```python
from build123d import *

# Parameters (mm, degrees)
RISER_DEPTH             = 7
SKETCH2_R               = 1.575
MOUNTING_HOLES_DEPTH    = 24.216373532
SKETCH3_W               = 40.15
SKETCH3_H               = 5.15
RECESS_DEPTH            = 3
FLANGE_DEPTH            = 7
SKETCH5_W               = 13.594480272
SKETCH5_H               = 6.925
FLANGE_CUTOUT_DEPTH     = 5
ANGLE_CUTOUT_DEPTH      = 32.901199964
ANGLE_CUTOUT_DEPTH_BACK = 32.901199964
FLANGE_CHAMFER_SIZE     = 1


with BuildPart() as part:
    # Sketch1 → Riser (new body)
    with BuildSketch(Plane(origin=(0, 0, 0), x_dir=(1, 0, 0), z_dir=(0, 1, 0))):
        Polygon((-18.999581839, 7), (18.999581839, 7), (21, 5.75), (21, 0), (-21, 0), (-21, 5.75), align=None)
    extrude(amount=RISER_DEPTH)

    # Sketch2 → Mounting Holes (cut, through all)
    with BuildSketch(Plane.XZ):
        with Locations(Location((16, -3.5, 0), (0, 0, 270))):
            Circle(SKETCH2_R)
        with Locations(Location((-16, -3.5, 0), (0, 0, 90))):
            Circle(SKETCH2_R)
    extrude(amount=-MOUNTING_HOLES_DEPTH, mode=Mode.SUBTRACT)

    # Sketch3 → Recess (cut)
    with BuildSketch(Plane(origin=(0, 7, 0), x_dir=(1, 0, 0), z_dir=(0, 1, 0))):
        with Locations((0, 3.5)):
            Rectangle(SKETCH3_W, SKETCH3_H)
    extrude(amount=-RECESS_DEPTH, mode=Mode.SUBTRACT)

    # Sketch4 → Flange (add)
    with BuildSketch(Plane(origin=(0, 0, 0), x_dir=(1, 0, 0), z_dir=(0, 1, 0))):
        Polygon((-18.999581839, 7), (18.999581839, 7), (7.797240136, 14), (-7.797240136, 14), align=None)
    extrude(amount=FLANGE_DEPTH)

    # Sketch5 → Flange Cutout (cut)
    with BuildSketch(Plane(origin=(0, 7, 0), x_dir=(1, 0, 0), z_dir=(0, 1, 0))):
        with Locations((0, 10.5375)):
            Rectangle(SKETCH5_W, SKETCH5_H)
        Polygon((-18.879556749, 7.075), (-7.797240136, 7.075), (-7.797240136, 14), align=None)
        Polygon((7.797240136, 7.075), (7.797240136, 14), (18.879556749, 7.075), align=None)
    extrude(amount=-FLANGE_CUTOUT_DEPTH, mode=Mode.SUBTRACT)

    # Sketch7 → Angle Cutout (cut, two sides: drawn at the far end of the back side and taken through both)
    with BuildSketch(Plane.ZY.offset(-6.797240136).offset(-ANGLE_CUTOUT_DEPTH_BACK)):
        Polygon((-7.075, 7), (-14, 2), (-14, 7), align=None)
    extrude(amount=ANGLE_CUTOUT_DEPTH + ANGLE_CUTOUT_DEPTH_BACK, mode=Mode.SUBTRACT)

    # Flange Chamfer
    flange_chamfer_edges = [part.edges().sort_by_distance(p)[0] for p in [
        (13.338398442, 2, -7.075),
        (-13.338398442, 2, -7.075),
        (0, 2, -7.075),
    ]]
    chamfer(flange_chamfer_edges, length=FLANGE_CHAMFER_SIZE)


solid = part.part
```
Verification items for the finished model (mm, model axes). A direction names the side the tool comes from. Give positions to 0.01 mm unless a question says otherwise; leave off trailing zeros. Loops run counter-clockwise (first coordinate to the right, second up) from the corner with the lowest first, then second, coordinate; pieces in that order, holes last. Notation, with made-up numbers: M 18.5,63 L 25.5,63 A26 cw 25.5,96 Z; hole C 59,48.25 d1. An arc over 180 degrees is marked long. Return JSON: item names as keys, results as strings.
1) Section check A-A, the plane y = 6. Enter the section's corners in (x, z) (3 decimals), and give its area (3 significant figures).
Findings:
{"outline": "M -21,-5.75 L -18.88,-7.075 L -7.797,-7.075 L -7.797,-8.46 L -6.797,-8.46 L -6.797,-7.075 L 6.797,-7.075 L 6.797,-8.46 L 7.797,-8.46 L 7.797,-7.075 L 18.88,-7.075 L 21,-5.75 L 21,0 L -21,0 Z; hole M -20.075,-6.075 L 20.075,-6.075 L 20.075,-0.925 L -20.075,-0.925 Z", "area": "90.3 mm2"}
2) Gauge pin test, flat ends, axial feed: P1, Ø2.5, axis at y = 3.5, z = -11, coming from the +X side; P2, Ø4, axis at y = 3.5, z = -11, coming from the -X side; P3, Ø4.5, axis at x = 0, z = -11, coming from the +Y side. Record the tip position at first contact, or that the pin passes through.
Findings:
{"P1": "stops at x = 7.8", "P2": "stops at x = -14.72", "P3": "stops at y = 2"}
3) Section check B-B, the plane z = -3.5. Enter the section's corners in (x, y) (3 decimals), and give its area (3 significant figures).
Findings:
{"outline": "M -21,0 L -17.575,0 L -17.575,4 L -20.075,4 L -20.075,7 L -21,7 Z; M -14.425,0 L 14.425,0 L 14.425,4 L -14.425,4 Z; M 17.575,0 L 21,0 L 21,7 L 20.075,7 L 20.075,4 L 17.575,4 Z", "area": "148 mm2"}
4) Section check C-C, the plane x = 5.5. Enter the section's corners in (y, z) (3 decimals), and give its area (3 significant figures).
Findings:
{"outline": "M 0,-14 L 2,-14 L 2,-8.075 L 3,-7.075 L 7,-7.075 L 7,-6.075 L 4,-6.075 L 4,-0.925 L 7,-0.925 L 7,0 L 0,0 Z", "area": "48.4 mm2"}
5) Section check D-D, the plane x = -16. Enter the section's corners in (y, z) (3 decimals), and give its area (3 significant figures).
Findings:
{"outline": "M 0,-8.874 L 2,-8.874 L 2,-8.075 L 3,-7.075 L 7,-7.075 L 7,-6.075 L 4,-6.075 L 4,-5.075 L 0,-5.075 Z; M 0,-1.925 L 4,-1.925 L 4,-0.925 L 7,-0.925 L 7,0 L 0,0 Z", "area": "25.6 mm2"}
6) Tool access check on faces 4 (the flat face through (0, 6, -6.075)), 5 (the flat face through (0, 5, -7.075)), 6 (the flat face through (-10, 2, -10)), 7 (the flat face through (10, 2, -10)). Record the directions out of +Z, -Z, +X, -X, +Y, -Y that give a thin tool (end or side, any length) a straight path to the whole face; none if there is none.
Findings:
{"face 4": "+Y", "face 5": "-Z, +Y", "face 6": "-Z, -X, +Y", "face 7": "-Z, +X, +Y"}
7) Mould release check, pull along Z, two halves, no side actions. Record for faces 1 (the flat face through (0, 3, 0)), 2 (the cylindrical face through (14.462, 1.972, -3.159)), 3 (the flat face through (-13.416, 2.493, -7.582)): released by +Z, released by -Z, zero draft, split by the parting line, or undercut.
Findings:
{"face 1": "released by +Z", "face 2": "undercut", "face 3": "released by -Z"}
8) Material ranges on L1, parallel to X at y = 1.75, z = -3.5 (3 decimals); L2, parallel to X at y = 3, z = -7.25; L3, parallel to Z at x = -16, y = 3.1 (3 decimals), recorded low to high. Write a range as [from, to].
Findings:
{"L1": "x = [-21, -17.575], [-14.425, 14.425], [17.575, 21]", "L2": "x = [-7.8, -6.8], [6.8, 7.8]", "L3": "z = [-7.075, -5.075], [-1.925, 0]"}
